from build123d import *

# Parameters (mm, degrees)
F0_R     = 10
F1_DEPTH = 200
F3_R     = 10
F3_R_2   = 8
F4_DEPTH = 5
F6_DEPTH = 15


with BuildPart() as f1:
    # F0 (on Front) → F1 (new body)
    with BuildSketch(Plane.XZ):
        Circle(F0_R)
    extrude(amount=F1_DEPTH)

    # F3 (on offset) → F4 (cut)
    with BuildSketch(Plane.XZ.offset(30)):
        Circle(F3_R)
        Circle(F3_R_2, mode=Mode.SUBTRACT)
    extrude(amount=F4_DEPTH, mode=Mode.SUBTRACT)

    # F5 (on face) → F6 (join)
    with BuildSketch(Plane(origin=(0, 0, 0), x_dir=(-1, 0, 0), z_dir=(0, 1, 0))):
        Polygon((16, -9.237604), (16, 9.237604), (0, 18.475209), (-16, 9.237604), (-16, -9.237604), (0, -18.475209), align=None)
    extrude(amount=F6_DEPTH)


solid = f1.part
Design review of the part built by this model. Coordinates are the model's own, in mm. A direction names the side the tool comes from. Coordinates: 2 decimals unless noted, no trailing zeros. Order: outer loops, then holes, each group sorted by start corner. A loop starts at its lowest first (then second) coordinate and runs counter-clockwise, first axis right, second up. Notation, with made-up numbers: (65, -10.5) -> (96, -10.5) arc R12 cw to (96, 9.5) -> close; hole circle Ø7 at (-8.75, -23). An arc over 180 degrees is marked (long way). Use one line per item in the form item = value. Start each with the question number.
(1) Add section D-D on z = -12.5. State the section outline as (x, y) points.
(2) The part is to be moulded in two halves that separate along Y. For faces 4 (the flat face through (-16, 7, 0)), 5 (the flat face through (0, -30, 8.2)), 6 (the flat face through (0, -35, 8.2)), 7 (the flat face through (0, -200, 0)), say which applies: +Y half, -Y half, draft (parallel to the pull), parting line (faces both ways), or undercut.
(3) Add section B-B on x = 3. State the section outline as (y, z) points, plus the area to 3 significant figures.
(4) For probe 1 along Y at (x, z) = (4, -8.5); probe 2 along Y at (x, z) = (7, -13.5); probe 3 along Z at (x, y) = (3.5, -103), list the stretches that pass through material, from the lowest coordinate up.
(5) Add section A-A on z = 0. State the section outline as (x, y) points.
(6) Insertion check: pin 1 (12 mm diameter, centred on x = -0.5, y = -85.5, fed in from +Z); pin 2 (8 mm diameter, centred on x = -2.5, z = 14, fed in from -Y); pin 3 (5 mm diameter, centred on y = -99.5, z = -6.5, fed in from +X). Each pin has a flat end and moves straight along its axis. Give the tip position at first contact, or say it passes through.
(7) For faces 1 (the cylindrical face through (-1.73, -32.47, -7.81)), 2 (the cylindrical face through (-2.17, -14.79, -9.76)), 3 (the flat face through (8.1, 7.4, -13.8)), list the 3-axis set-ups (+Z, -Z, +X, -X, +Y, -Y) from which the entire face can be reached by the end or side of a thin tool; tool diameter is ignored.
(8) Add section C-C on y = -161. State the section outline as (x, z) points, plus the area to 3 significant figures.
Answer block:
q1.outline = (-10.35, 0) -> (10.35, 0) -> (10.35, 15) -> (-10.35, 15) -> close
q2.face_4 = draft
q2.face_5 = undercut
q2.face_6 = undercut
q2.face_7 = -Y half
q3.outline = (-200, -9.54) -> (-35, -9.54) -> (-35, -7.42) -> (-30, -7.42) -> (-30, -9.54) -> (0, -9.54) -> (0, -16.74) -> (15, -16.74) -> (15, 16.74) -> (0, 16.74) -> (0, 9.54) -> (-30, 9.54) -> (-30, 7.42) -> (-35, 7.42) -> (-35, 9.54) -> (-200, 9.54) -> close
q3.area = 4,300 mm²
q4.probe_1 = -200 to -35, -30 to 15
q4.probe_2 = 0 to 15
q4.probe_3 = -9.37 to 9.37
q5.outline = (-16, 0) -> (-10, 0) -> (-10, -30) -> (-8, -30) -> (-8, -35) -> (-10, -35) -> (-10, -200) -> (10, -200) -> (10, -35) -> (8, -35) -> (8, -30) -> (10, -30) -> (10, 0) -> (16, 0) -> (16, 15) -> (-16, 15) -> close
q6.pin_1 = 10
q6.pin_2 = 0
q6.pin_3 = 9.17
q7.face_1 = none
q7.face_2 = -Y
q7.face_3 = -Z, +X, +Y, -Y
q8.outline = circle Ø20 at (0, 0)
q8.area = 314 mm²
